The listing builds one solid part. Answer for the finished solid, in the listing's coordinates (mm). Face numbers are marked on the shaded views. A direction names the side the tool comes from. Give positions to 0.01 mm unless a question says otherwise; leave off trailing zeros. Order: outer loops, then holes, each group sorted by start corner. A loop starts at its lowest first (then second) coordinate and runs counter-clockwise, first axis right, second up. Notation, with made-up numbers: (88.25, 23.5) - (106.25, 23.5) arc R21 cw to (106.25, 55.5) - close; hole circle Ø3 at (7.25, 32). An arc over 180 degrees is marked (long way). Answer as a JSON object with one key per item and string values. Group by question number.
Q1. A cutting plane is placed at A-A, the plane z = 0.8. Count the separate pieces of the cut face and the enclosed holes in it, and give its area (3 significant figures).
Q2. Consider line 1 (Z direction, x = -6, y = 2.4); line 2 (X direction, y = 1.2, z = 0.8); line 3 (X direction, y = 2.25, z = 0.8). Determine where each line is inside the solid, lowest interval first.
Q3. A cutting plane is placed at C-C, the plane x = -0.75. Give the vertices of the cut face in (y, z), and give its area (3 significant figures).
Q4. Given pin 1 (3 mm diameter, centred on x = 0, z = 0, fed in from -Y), flat-ended and moving along its own axis, determine where the tip first touches the part or whether it passes through.
Q5. The mould has two halves that part along X. Classify the marked faces 1, 2 and 3: released by +X, released by -X, zero draft, split by the parting line, or undercut.
Q6. For the marked faces 4 and 5, determine the directions among +Z, -Z, +X, -X, +Y, -Y from which every point of the face is accessible in a straight line to the end or side of a thin tool.
Autodesk Inventor part; units mm, degrees
ref_plane "YZ Plane" through (0, 0, 0) normal (1, 0, 0) x (0, 1, 0)
ref_plane "XZ Plane" through (0, 0, 0) normal (0, 1, 0) x (-1, 0, 0)
ref_plane "XY Plane" through (0, 0, 0) normal (0, 0, 1) x (1, 0, 0)
sketch "Skizze1" plane through (0, 0, 0) normal (0, 1, 0) x (-1, 0, 0)
  line L0 (8.5, -3) -> (-8.5, -3)
  line L1 (-8.5, -3) -> (-8.5, 3)
  line L2 (-8.5, 3) -> (8.5, 3)
  line L3 (8.5, 3) -> (8.5, -3)
  line L4 (8.5, -3) -> (-8.5, 3) construction
  line L5 (-8.5, -3) -> (8.5, 3) construction
  point P0 (0, 0)
  dimension "d0" = 17
  dimension "d1" = 6
extrude "Extrusion1" add sketch "Skizze1" along normal blind 4
sketch "Skizze2" plane through (0, 0, 0) normal (0, -1, 0) x (1, 0, 0)
  line L0 (-11.9, 0) -> (11.9, 0)
  line L1 (0, 4.2) -> (0, -4.2)
  point P0 (0, 0)
  point P1 (-6, 0.8)
  point P2 (6, 0.8)
  dimension "d5" = 0.8
  dimension "d6" = 6
hole "Bohrung1" at (-6, 0, 0.8) at (6, 0, 0.8) direction (0, 1, 0) diameter 1.9 end through all
sketch "Skizze5" plane through (0, 0, 0) normal (0, -1, 0) x (1, 0, 0)
  line L0 (8.5, -3) -> (-8.5, -3)
  line L1 (8.5, 3) -> (8.5, -3)
  line L2 (-8.5, -3) -> (8.5, -3)
  line L3 (8.5, -3) -> (8.5, -2)
  line L4 (8.5, -2) -> (-8.5, -2)
  line L5 (-8.5, -2) -> (-8.5, -3)
  point P0 (0, 0)
  dimension "d29" = 1
extrude "Extrusion4" [suppressed]
sketch "Skizze6" plane through (0, 0, 0) normal (0, -1, 0) x (1, 0, 0)
  line L0 (8.5, -3) -> (8.5, 3)
  line L1 (8.5, 3) -> (-8.5, 3)
  line L2 (-8.5, 3) -> (-8.5, -3)
  circle A0 centre (-6, 0.8) radius 0.95
  circle A1 centre (6, 0.8) radius 0.95
  line L3 (8.5, 3) -> (-8.5, 3)
  line L4 (-3, 3) -> (3, 3)
  line L5 (3, 3) -> (3, -2)
  line L6 (3, -2) -> (-3, -2)
  line L7 (-3, -2) -> (-3, 3)
  line L8 (0, 4.2) -> (0, -4.2)
  line L9 (-8.5, -3) -> (8.5, -3)
  point P0 (0, 0)
  point P1 (0, 3)
  dimension "d32" = 6
extrude "Extrusion5" cut sketch "Skizze6" against normal through all contours L5 L6 L8 L1 | L6 L7 L1 L8
sketch "Skizze7" plane through (-8.5, -2, -2) normal (0, 0, 1) x (1, 0, 0)
  line L0 (0, 0) -> (1, 0)
  line L1 (1, 0) -> (1, 2)
  line L2 (1, 2) -> (0, 2)
  line L3 (0, 2) -> (0, 0)
  line L4 (17, 0) -> (0, 0)
  line L5 (11.5, 2) -> (17, 2)
  line L6 (17, 0) -> (16, 0)
  line L7 (16, 0) -> (16, 2)
  line L8 (16, 2) -> (17, 2)
  line L9 (17, 2) -> (17, 0)
  point P0 (8.5, 2)
  dimension "d35" = 1
  dimension "d36" = 1
extrude "Extrusion6" [suppressed]
chamfer "Fase4" [suppressed]
chamfer "Fase6" distance 1.5 distance2 4 1 edges at (-3, 0, 0.5) measured on face at (1, 0, -2.6667)
chamfer "Fase7" distance 1.5 distance2 4 1 edges at (3, 0, 0.5) measured on face at (-1, 0, -2.6667)
fillet "Rundung3" radius 2 4 edges at (-3.7498, 1.9998, 3) (-3, 3.9998, 3) (3.7497, 1.9997, 3) (3, 3.9997, 3)
sketch "Skizze8" plane through (0, 0, 0) normal (0, -1, 0) x (1, 0, 0)
  line L0 (-3, 3) -> (-7.5, 3)
  line L1 (-7.5, 3) -> (-7.5, -2)
  line L2 (-7.5, -2) -> (-3, -2)
  line L3 (-3, -2) -> (-3, 3)
  circle A0 centre (-6, 1) radius 0.95
  line L4 (3, 3) -> (3, -2)
  line L5 (3, -2) -> (7.5, -2)
  line L6 (7.5, -2) -> (7.5, 3)
  line L7 (7.5, 3) -> (3, 3)
  circle A1 centre (6, 1) radius 0.95
  line L8 (-7.5, 3) -> (-7.5, -2)
  line L9 (-7.5, -2) -> (-3, -2)
  line L10 (-3, -2) -> (-3, 3)
  line L11 (-3, 3) -> (-7.5, 3)
  line L12 (7.5, -2) -> (7.5, 3)
  line L13 (3, 3) -> (3, -2)
  line L14 (3, -2) -> (7.5, -2)
  line L15 (7.5, 3) -> (3, 3)
properties part number "LED Schirm"
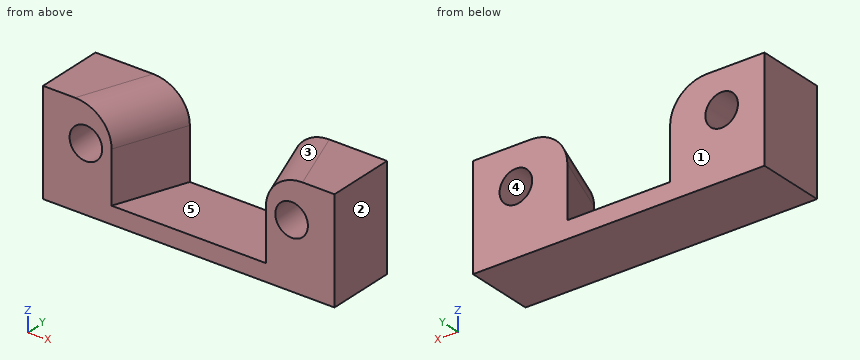
Reply:
{
 "1": {"separate pieces": "4", "enclosed holes": "0", "area": "22.8 mm^2"},
 "2": {"line 1": "z = -3 to -0.15, 1.75 to 3", "line 2": "x = -8.5 to -6.95, -5.05 to -4.05, 4.05 to 5.05, 6.95 to 8.5", "line 3": "x = -8.5 to -6.95, -5.05 to -3.66, 3.66 to 5.05, 6.95 to 8.5"},
 "3": {"outline": "(0, -3) - (4, -3) - (4, -2) - (0, -2) - close", "area": "4.00 mm^2"},
 "4": {"pin 1": "passes through"},
 "5": {"face 1": "zero draft", "face 2": "released by +X", "face 3": "undercut"},
 "6": {"face 4": "+Y, -Y", "face 5": "+Z, -Y"}
}
